```python
from build123d import *

# Parameters (mm, degrees)
F0_W     = 528.32
F0_H     = 381
F1_DEPTH = 50.8
F2_W     = 515.62
F2_H     = 368.3
F3_DEPTH = 50.165
F4_W     = 72.005392
F4_H     = 25.4
F5_DEPTH = 6.35
F6_R     = 11.43


with BuildPart() as f1:
    # F0 (on Top) → F1 (new body)
    with BuildSketch(Plane.XY):
        Rectangle(F0_W, F0_H)
    extrude(amount=F1_DEPTH)

    # F2 (on face) → F3 (cut)
    with BuildSketch(Plane.XY.offset(50.8)):
        Rectangle(F2_W, F2_H)
    extrude(amount=-F3_DEPTH, mode=Mode.SUBTRACT)

    # F4 (on face) → F5 (cut)
    with BuildSketch(Plane.YZ.offset(264.16)):
        with Locations((-1.279233, 25.4)):
            Rectangle(F4_W, F4_H)
    extrude(amount=-F5_DEPTH, mode=Mode.SUBTRACT)

    # F6
    f6_edges = [f1.edges().sort_by_distance(p)[0] for p in [
        (260.985, 34.723463, 12.7),
        (260.985, -37.281929, 12.7),
        (260.985, -37.281929, 38.1),
        (260.985, 34.723463, 38.1),
    ]]
    fillet(f6_edges, radius=F6_R)


solid = f1.part
```
Here's how the part is built. I have some questions about the finished solid (model axes, mm). A direction names the side the tool comes from. Coordinates: 2 decimals unless noted, no trailing zeros. Order: outer loops, then holes, each group sorted by start corner. A loop starts at its lowest first (then second) coordinate and runs counter-clockwise, first axis right, second up.
1) Imagine slicing it at C-C on x = 211. List the corners of the cut face in (y, z) for me (3 decimals), and give its area (3 significant figures).
2) We'd pull the mould along X, two halves only. Please class faces 4 (the face through (-264.16, -3, 25)), 5 (the face through (257.81, -3, 9)), 6 (the face through (260.941, -34.023, 16.137)): +X half, -X half, draft (parallel to the pull), parting line (faces both ways), or undercut.
3) Imagine slicing it at A-A on z = 6. List the corners of the cut face in (x, y) for me, and give its area (3 significant figures).
4) Imagine slicing it at B-B on y = 120. List the corners of the cut face in (x, z) for me (3 decimals), and give its area (3 significant figures).
5) Which directions (+Z, -Z, +X, -X, +Y, -Y) give clear straight access to the entire face, cutting with the end or side of a thin tool? Please do faces 1 (the face through (-4, -184.15, 26)), 2 (the face through (260.941, -34.023, 34.663)), 3 (the face through (264.16, -3, 42)).
6) Will this pin go through, and if not, where does the flat tip stop? pin 1 (4 mm diameter, centred on x = 114, y = 104, fed in from +Z) (3 decimals).
7) I need wall thicknesses on line 1 (Y direction, x = 223.5, z = 23.5); line 2 (X direction, y = -71.5, z = 16.5); line 3 (Z direction, x = -17, y = 156) (3 decimals). Which ranges of each line are inside material? Lowest first, please.
Response values:
1. outline: (-190.5, 0) - (190.5, 0) - (190.5, 50.8) - (184.15, 50.8) - (184.15, 0.635) - (-184.15, 0.635) - (-184.15, 50.8) - (-190.5, 50.8) - close
1. area: 879 mm2
2. face 4: -X half
2. face 5: undercut
2. face 6: draft
3. outline: (-264.16, -190.5) - (264.16, -190.5) - (264.16, 190.5) - (-264.16, 190.5) - close; hole (-257.81, -184.15) - (257.81, -184.15) - (257.81, 184.15) - (-257.81, 184.15) - close
3. area: 11,400 mm2
4. outline: (-264.16, 0) - (264.16, 0) - (264.16, 50.8) - (257.81, 50.8) - (257.81, 0.635) - (-257.81, 0.635) - (-257.81, 50.8) - (-264.16, 50.8) - close
4. area: 973 mm2
5. face 1: +Z
5. face 2: +X
5. face 3: +Z, -Z, +X, +Y, -Y
6. pin 1: stops at z = 0.635
7. line 1: y = -190.5 to -184.15, 184.15 to 190.5
7. line 2: x = -264.16 to -257.81, 257.81 to 264.16
7. line 3: z = 0 to 0.635
